The figure shows three views and two pictorial views of one solid part (mm, origin at its lowest corner). Answer the questions. A direction names the side the tool comes from. Round coordinates to 2 decimals unless told otherwise and drop trailing zeros. Order: outer loops, then holes, each group sorted by start corner. A loop starts at its lowest first (then second) coordinate and runs counter-clockwise, first axis right, second up. Notation, with made-up numbers: (50.25, 57) -> (63.25, 57) arc R35 cw to (63.25, 93) -> close; hole circle Ø1 at (75, 48.5). An arc over 180 degrees is marked (long way). One line per item, written item: value. Start each with the question number.
1. The mould has two halves that part along X. Classify the marked faces 3, 4 and 5: released by +X, released by -X, zero draft, split by the parting line, or undercut.
2. Section C-C (y = 23) is taken. Give the vertices of the cut face in (x, z), then the cut area to 3 significant figures.
3. Consider line 1 (Y direction, x = 25, z = 0.4); line 2 (X direction, y = 23, z = 2.35) (1 decimal); line 3 (X direction, y = 22, z = 3.35). Determine where each line is inside the solid, lowest interval first.
4. Flat-ended cylindrical pins translate along their axes: pin 1 Ø5 at (x, y) = (10.5, 21.5) entering from -Z; pin 2 Ø2.5 at (x, z) = (25, 2) entering from -Y; pin 3 Ø2 at (x, z) = (38, 1) entering from +Y; pin 4 Ø1.5 at (y, z) = (32, 4) entering from -X. Find the tip coordinate at first contact, or state that the pin passes through.
5. Section B-B (z = 3.95) is taken. Give the vertices of the cut face in (x, y), then the cut area to 3 significant figures.
6. For the marked faces 1 and 2, determine the directions among +Z, -Z, +X, -X, +Y, -Y from which every point of the face is accessible in a straight line to the end or side of a thin tool.
7. Section D-D (y = 5.5) is taken. Give the vertices of the cut face in (x, z) (1 decimal).
8. Section A-A (x = 25.4) is taken. Give the vertices of the cut face in (y, z).
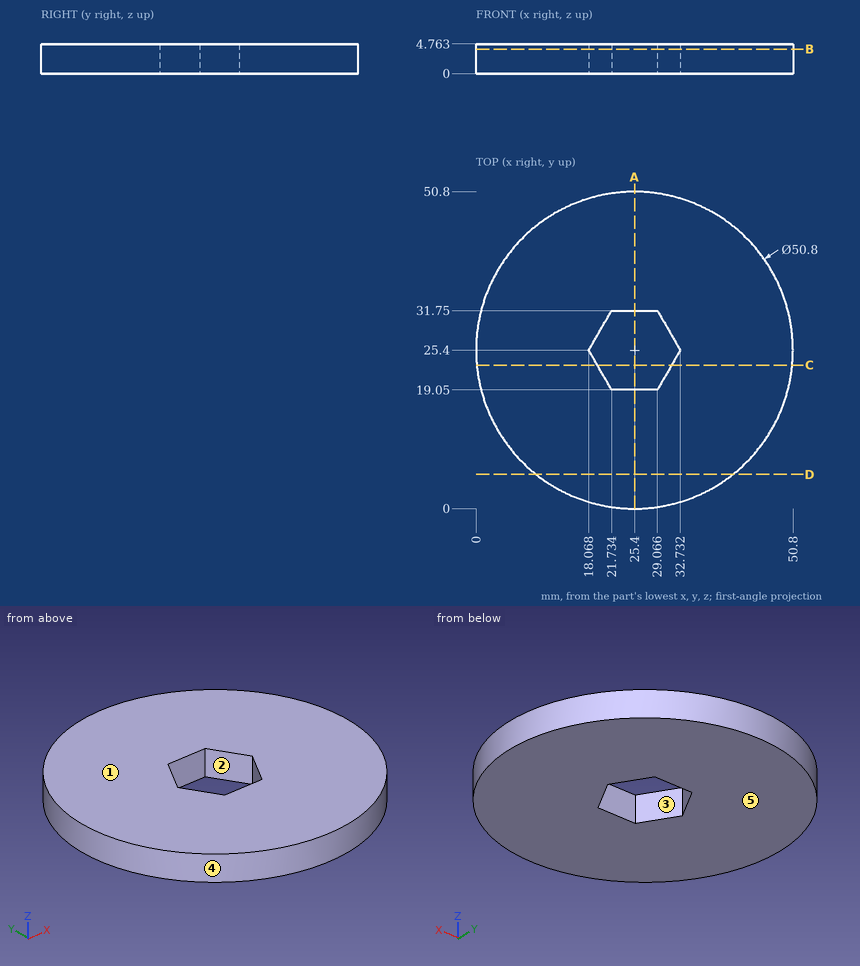
Answer:
1. face 3: undercut
1. face 4: split by the parting line
1. face 5: zero draft
2. outline: (0.11, 0) -> (19.45, 0) -> (19.45, 4.76) -> (0.11, 4.76) -> close; (31.35, 0) -> (50.69, 0) -> (50.69, 4.76) -> (31.35, 4.76) -> close
2. area: 184 mm^2
3. line 1: 0 to 19.05, 31.75 to 50.8
3. line 2: 0.1 to 19.5, 31.3 to 50.7
3. line 3: 0.23 to 20.03, 30.77 to 50.57
4. pin 1: z = 0
4. pin 2: y = 0
4. pin 3: y = 48
4. pin 4: x = 0.68
5. outline: circle Ø50.8 at (25.4, 25.4); hole (18.07, 25.4) -> (21.73, 19.05) -> (29.07, 19.05) -> (32.73, 25.4) -> (29.07, 31.75) -> (21.73, 31.75) -> close
5. area: 1,890 mm^2
6. face 1: +Z, +X, -X, +Y, -Y
6. face 2: +Z, -Z
7. outline: (9.6, 0) -> (41.2, 0) -> (41.2, 4.8) -> (9.6, 4.8) -> close
8. outline: (0, 0) -> (19.05, 0) -> (19.05, 4.76) -> (0, 4.76) -> close; (31.75, 0) -> (50.8, 0) -> (50.8, 4.76) -> (31.75, 4.76) -> close
